from build123d import *

# Parameters (mm, degrees)
SKETCH_W        = 100
SKETCH_H        = 64
SKETCH_R        = 5
SKETCH_R_2      = 3.2
SKETCH_R_3      = 4
PAD_DEPTH       = 15
SKETCH001_R     = 11.02
POCKET_DEPTH    = 7.2
SKETCH002_R     = 6
POCKET001_DEPTH = 7


with BuildPart() as part:
    # Sketch → Pad (new body)
    with BuildSketch(Plane.XY):
        with Locations((50, 32)):
            Rectangle(SKETCH_W, SKETCH_H)
        with Locations((50, 42.85)):
            Circle(SKETCH_R, mode=Mode.SUBTRACT)
        with Locations((20, 10)):
            Circle(SKETCH_R_2, mode=Mode.SUBTRACT)
        with Locations((80, 10)):
            Circle(SKETCH_R_2, mode=Mode.SUBTRACT)
        with Locations((82, 42.85)):
            Circle(SKETCH_R_3, mode=Mode.SUBTRACT)
        with Locations((18, 42.85)):
            Circle(SKETCH_R_3, mode=Mode.SUBTRACT)
    extrude(amount=PAD_DEPTH)

    # Sketch001 (on Face11 of Pad) → Pocket (cut)
    with BuildSketch(Plane.XY.offset(15)):
        with Locations((50, 42.85)):
            Circle(SKETCH001_R)
    extrude(amount=-POCKET_DEPTH, mode=Mode.SUBTRACT)

    # Sketch002 (on Face4 of Pocket) → Pocket001 (cut)
    with BuildSketch(Plane(origin=(0, 0, 0), x_dir=(1, 0, 0), z_dir=(0, 0, -1))):
        with Locations((20, -10)):
            Circle(SKETCH002_R)
        with Locations((80, -10)):
            Circle(SKETCH002_R)
    extrude(amount=-POCKET001_DEPTH, mode=Mode.SUBTRACT)


solid = part.part
Here's how the part is built. I have some questions about the finished solid (model axes, mm). A direction names the side the tool comes from. Round coordinates to 2 decimals unless told otherwise and drop trailing zeros. Loops run counter-clockwise (first coordinate to the right, second up) from the corner with the lowest first, then second, coordinate; pieces in that order, holes last. Notation, with made-up numbers: (-23, 6.5) - (3, 6.5) arc R21 cw to (3, 43.5) - close; hole circle Ø8 at (35, 32.5). An arc over 180 degrees is marked (long way). One line per question, with ' | ' between items. Start each with the question number.
Q1. I want a section at A-A (y = 10). Write out the boundary of the cut face in (x, z), then the cut area to 3 significant figures.
Q2. Will these pins go through, and if not, where does the flat tip stop? pin 1 (5 mm diameter, centred on x = 80, y = 10, fed in from +Z); pin 2 (6 mm diameter, centred on x = 79, y = 9.5, fed in from -Z); pin 3 (11 mm diameter, centred on x = 49, y = 39, fed in from +Z).
Q3. I want a section at B-B (z = 5.5). Write out the boundary of the cut face in (x, y), then the cut area to 3 significant figures.
Q4. I want a section at D-D (y = 42.85). Write out the boundary of the cut face in (x, z), then the cut area to 3 significant figures.
Q5. I want a section at C-C (x = 50). Write out the boundary of the cut face in (y, z), then the cut area to 3 significant figures.
Q6. Please list where these lines run through material, in increasing order: line 1 (X direction, y = 10, z = 13); line 2 (X direction, y = 10, z = 2.75); line 3 (Y direction, x = 80, z = 13). Write a range as [from, to].
Q7. We'd pull the mould along X, two halves only. Please class faces 4 (the flat face through (0, 32, 7)), 5 (the flat face through (100, 32, 7)), 6 (the cylindrical face through (46.03, 39.81, 3.85)): +X half, -X half, draft (parallel to the pull), parting line (faces both ways), or undercut.
Q8. For faces 1 (the flat face through (83, 13, 7)), 2 (the flat face through (55, 41, 7.8)), 3 (the flat face through (49, 25, 15)), which set-ups out of +Z, -Z, +X, -X, +Y, -Y let a thin tool reach every point of the face, with its end or its side?
Response values:
1) outline: (0, 0) - (14, 0) - (14, 7) - (16.8, 7) - (16.8, 15) - (0, 15) - close; (23.2, 7) - (26, 7) - (26, 0) - (74, 0) - (74, 7) - (76.8, 7) - (76.8, 15) - (23.2, 15) - close; (83.2, 7) - (86, 7) - (86, 0) - (100, 0) - (100, 15) - (83.2, 15) - close | area: 1,230 mm²
2) pin 1: passes through | pin 2: stops at z = 7 | pin 3: stops at z = 7.8
3) outline: (0, 0) - (100, 0) - (100, 64) - (0, 64) - close; hole circle Ø12 at (20, 10); hole circle Ø8 at (18, 42.85); hole circle Ø10 at (50, 42.85); hole circle Ø12 at (80, 10); hole circle Ø8 at (82, 42.85) | area: 5,990 mm²
4) outline: (0, 0) - (14, 0) - (14, 15) - (0, 15) - close; (22, 0) - (45, 0) - (45, 7.8) - (38.98, 7.8) - (38.98, 15) - (22, 15) - close; (55, 0) - (78, 0) - (78, 15) - (61.02, 15) - (61.02, 7.8) - (55, 7.8) - close; (86, 0) - (100, 0) - (100, 15) - (86, 15) - close | area: 1,020 mm²
5) outline: (0, 0) - (37.85, 0) - (37.85, 7.8) - (31.83, 7.8) - (31.83, 15) - (0, 15) - close; (47.85, 0) - (64, 0) - (64, 15) - (53.87, 15) - (53.87, 7.8) - (47.85, 7.8) - close | area: 723 mm²
6) line 1: x = [0, 16.8], [23.2, 76.8], [83.2, 100] | line 2: x = [0, 14], [26, 74], [86, 100] | line 3: y = [0, 6.8], [13.2, 39.39], [46.31, 64]
7) face 4: -X half | face 5: +X half | face 6: undercut
8) face 1: -Z | face 2: +Z | face 3: +Z, +X, -X, +Y, -Y
